Here's how the part is built. I have some questions about the finished solid (model axes, mm). Face numbers are marked on the shaded views. A direction names the side the tool comes from. Round coordinates to 2 decimals unless told otherwise and drop trailing zeros. Write each loop counter-clockwise with the first axis right and the second up, starting at its lowest first coordinate (ties: lowest second). Pieces come first, ordered by that corner, then holes. Notation, with made-up numbers: (-27.5, -27.75) -> (-11.5, -27.75) arc R27 ccw to (-11.5, -9.75) -> close; hole circle Ø1 at (47.25, 86.5). An arc over 180 degrees is marked (long way). Put each result on its own line as item: value. Start each with the question number.
1. Suppose I cut it at A-A (y = 0). Please give me the cut outline in (x, z).
2. Suppose I cut it at C-C (z = 8). Please give me the cut outline in (x, y), then the cut area to 3 significant figures.
3. Which directions (+Z, -Z, +X, -X, +Y, -Y) give clear straight access to the entire face, cutting with the end or side of a thin tool? Please do the marked faces 5, 6 and 7.
4. Suppose I cut it at D-D (y = 15). Please give me the cut outline in (x, z), then the cut area to 3 significant figures.
5. For pin 1 (5.5 mm diameter, centred on y = 16.5, z = 6.5, fed in from +X); pin 2 (6 mm diameter, centred on x = 1.5, z = 2, fed in from +Y); pin 3 (12 mm diameter, centred on x = -42, y = 0, fed in from +Z); pin 4 (2 mm diameter, centred on y = 0, z = -2, fed in from -X), each with a flat end and sliding along its axis, tell me the tip position at first contact or that it passes through.
6. We'd pull the mould along Y, two halves only. Please class the marked faces 1, 2, 3 and 4: +Y half, -Y half, draft (parallel to the pull), parting line (faces both ways), or undercut.
7. I need wall thicknesses on probe 1 along Y at (x, z) = (-18.5, 8); probe 2 along Y at (x, z) = (-42, -7.4); probe 3 along X at (y, z) = (-1, 1.25). Which ranges of each line are inside material? Lowest first, please. Write a range as from..to.
8. Suppose I cut it at B-B (x = -42). Please give me the cut outline in (y, z), then the cut area to 3 significant figures.
```python
from build123d import *

# Parameters (mm, degrees)
SKETCH_1_W      = 60
SKETCH_1_H      = 20
EXTRUDE_1_DEPTH = 10
SKETCH_2_R      = 7.5
EXTRUDE_2_DEPTH = 5


with BuildPart() as part:
    # 草图1 → 凸台-拉伸1 (new, symmetric)
    with BuildSketch(Plane.XY):
        Rectangle(SKETCH_1_W, SKETCH_1_H)
    extrude(amount=EXTRUDE_1_DEPTH, both=True)

    # 草图2 → 凸台-拉伸2 (add)
    with BuildSketch(Plane.XY.offset(-5)):
        with BuildLine():
            Line((-30, 20), (-30, -20))
            ThreePointArc((-30, -20), (-50, 0), (-30, 20))
        make_face()
        with Locations((-42, 0)):
            Circle(SKETCH_2_R, mode=Mode.SUBTRACT)
    extrude_2 = extrude(amount=-EXTRUDE_2_DEPTH)

    # 镜向4: 凸台-拉伸2 across plane
    add(extrude_2.mirror(Plane.XY))


solid = part.part
```
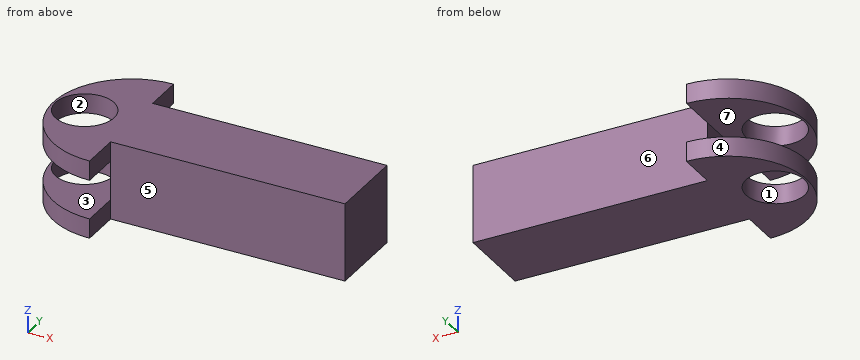
Verdict:
1. outline: (-50, -10) -> (-49.5, -10) -> (-49.5, -5) -> (-50, -5) -> close; (-50, 5) -> (-49.5, 5) -> (-49.5, 10) -> (-50, 10) -> close; (-34.5, -10) -> (30, -10) -> (30, 10) -> (-34.5, 10) -> (-34.5, 5) -> (-30, 5) -> (-30, -5) -> (-34.5, -5) -> close
2. outline: (-30, -20) -> (-30, -10) -> (30, -10) -> (30, 10) -> (-30, 10) -> (-30, 20) arc R20 ccw to start; hole circle Ø15 at (-42, 0)
2. area: 1,650 mm^2
3. face 5: +Z, -Z, +X, -Y
3. face 6: +Z, -Z, +X, +Y
3. face 7: -X, +Y, -Y
4. outline: (-43.23, -10) -> (-30, -10) -> (-30, -5) -> (-43.23, -5) -> close; (-43.23, 5) -> (-30, 5) -> (-30, 10) -> (-43.23, 10) -> close
4. area: 132 mm^2
5. pin 1: stops at x = -30
5. pin 2: stops at y = 10
5. pin 3: passes through
5. pin 4: stops at x = -30
6. face 1: undercut
6. face 2: undercut
6. face 3: draft
6. face 4: parting line
7. probe 1: y = -10..10
7. probe 2: y = -16..-7.5, 7.5..16
7. probe 3: x = -30..30
8. outline: (-16, -10) -> (-7.5, -10) -> (-7.5, -5) -> (-16, -5) -> close; (-16, 5) -> (-7.5, 5) -> (-7.5, 10) -> (-16, 10) -> close; (7.5, -10) -> (16, -10) -> (16, -5) -> (7.5, -5) -> close; (7.5, 5) -> (16, 5) -> (16, 10) -> (7.5, 10) -> close
8. area: 170 mm^2
